from build123d import *

# Parameters (mm, degrees)
AUFSATZ_LINEAR_AUSTRAGEN1_DEPTH = 113
AUFSATZ_LINEAR_START            = -1
SKIZZE1_4_R                     = 3
AUFSATZ_LINEAR_AUSTRAGEN2_DEPTH = 1
SCHNITT_LINEAR_AUSTRAGEN1_DEPTH = 1
SKIZZE3_W                       = 2.5
SKIZZE3_H                       = 11
SKIZZE3_W_2                     = 3.5
SKIZZE3_H_2                     = 6.5
SCHNITT_LINEAR_AUSTRAGEN2_DEPTH = 2


with BuildPart() as part:
    # Skizze1 → Aufsatz-Linear austragen1 (new body)
    with BuildSketch(Plane(origin=(0, 0, 0), x_dir=(1, 0, 0), z_dir=(0, 1, 0))):
        with BuildLine():
            Line((-15.125, 17.875), (15.125, 17.875))
            ThreePointArc((15.125, 17.875), (17.069543648, 17.069543648), (17.875, 15.125))
            Line((17.875, 15.125), (17.875, -15.125))
            ThreePointArc((17.875, -15.125), (17.069543648, -17.069543648), (15.125, -17.875))
            Line((15.125, -17.875), (-15.125, -17.875))
            ThreePointArc((-15.125, -17.875), (-17.069543648, -17.069543648), (-17.875, -15.125))
            Line((-17.875, -15.125), (-17.875, 15.125))
            ThreePointArc((-17.875, 15.125), (-17.069543648, 17.069543648), (-15.125, 17.875))
        make_face()
        with BuildLine():
            ThreePointArc((-15.125, 16.875), (-16.362436867, 16.362436867), (-16.875, 15.125))
            Line((-16.875, 15.125), (-16.875, -15.125))
            ThreePointArc((-16.875, -15.125), (-16.362436867, -16.362436867), (-15.125, -16.875))
            Line((-15.125, -16.875), (15.125, -16.875))
            ThreePointArc((15.125, -16.875), (16.362436867, -16.362436867), (16.875, -15.125))
            Line((16.875, -15.125), (16.875, 15.125))
            ThreePointArc((16.875, 15.125), (16.362436867, 16.362436867), (15.125, 16.875))
            Line((15.125, 16.875), (-15.125, 16.875))
        make_face(mode=Mode.SUBTRACT)
    extrude(amount=AUFSATZ_LINEAR_AUSTRAGEN1_DEPTH)

    # Skizze1_4 → Aufsatz-Linear austragen2 (add)
    with BuildSketch(Plane(origin=(0, 0, 0), x_dir=(1, 0, 0), z_dir=(0, 1, 0)).offset(AUFSATZ_LINEAR_START)):
        with BuildLine():
            Line((15.125, 17.875), (-15.125, 17.875))
            ThreePointArc((-15.125, 17.875), (-17.069543648, 17.069543648), (-17.875, 15.125))
            Line((-17.875, 15.125), (-17.875, -15.125))
            ThreePointArc((-17.875, -15.125), (-17.069543648, -17.069543648), (-15.125, -17.875))
            Line((-15.125, -17.875), (15.125, -17.875))
            ThreePointArc((15.125, -17.875), (17.069543648, -17.069543648), (17.875, -15.125))
            Line((17.875, -15.125), (17.875, 15.125))
            ThreePointArc((17.875, 15.125), (17.069543648, 17.069543648), (15.125, 17.875))
        make_face()
        with BuildLine():
            Line((-10, 8), (10, 8))
            ThreePointArc((10, 8), (11.414213562, 7.414213562), (12, 6))
            Line((12, 6), (12, 0))
            ThreePointArc((12, 0), (11.414213562, -1.414213562), (10, -2))
            Line((10, -2), (-10, -2))
            ThreePointArc((-10, -2), (-11.414213562, -1.414213562), (-12, 0))
            Line((-12, 0), (-12, 6))
            ThreePointArc((-12, 6), (-11.414213562, 7.414213562), (-10, 8))
        make_face(mode=Mode.SUBTRACT)
        with Locations(Location((0, -9.5, 0), (0, 0, 270))):
            Circle(SKIZZE1_4_R, mode=Mode.SUBTRACT)
    extrude(amount=AUFSATZ_LINEAR_AUSTRAGEN2_DEPTH)

    # Skizze2 → Schnitt-Linear austragen1 (cut)
    with BuildSketch(Plane.XY.offset(17.875)):
        with BuildLine():
            Line((-10.5, 38), (10.5, 38))
            ThreePointArc((10.5, 38), (11.914213562, 37.414213562), (12.5, 36))
            Line((12.5, 36), (12.5, 27))
            ThreePointArc((12.5, 27), (11.914213562, 25.585786438), (10.5, 25))
            Line((10.5, 25), (-10.5, 25))
            ThreePointArc((-10.5, 25), (-11.914213562, 25.585786438), (-12.5, 27))
            Line((-12.5, 27), (-12.5, 36))
            ThreePointArc((-12.5, 36), (-11.914213562, 37.414213562), (-10.5, 38))
        make_face()
    extrude(amount=-SCHNITT_LINEAR_AUSTRAGEN1_DEPTH, mode=Mode.SUBTRACT)

    # Skizze3 → Schnitt-Linear austragen2 (cut)
    with BuildSketch(Plane(origin=(17.875, 0, 0), x_dir=(0, 0, -1), z_dir=(1, 0, 0))):
        with Locations((12.25, 7.5)):
            Rectangle(SKIZZE3_W, SKIZZE3_H)
        with Locations((13.75, 20.25)):
            Rectangle(SKIZZE3_W_2, SKIZZE3_H_2)
    extrude(amount=-SCHNITT_LINEAR_AUSTRAGEN2_DEPTH, mode=Mode.SUBTRACT)


solid = part.part
Can you work these out from the model? Positions are in its coordinate system, mm. A direction names the side the tool comes from. Coordinates: 2 decimals unless noted, no trailing zeros. Write each loop counter-clockwise with the first axis right and the second up, starting at its lowest first coordinate (ties: lowest second). Pieces come first, ordered by that corner, then holes. Notation, with made-up numbers: M -10,10 L 2,10 A16 cw 2,36 Z; hole C 37,5.25 d10. An arc over 180 degrees is marked long. Use one line per item in the form item = value.
Q1. For P1, Ø7, axis at x = 0, z = 9.5, coming from the +Y side; P2, Ø1.1, axis at x = 17.5, y = 18.5, coming from the -Z side; P3, Ø0.5, axis at x = 17.5, y = 6, coming from the +Z side; P4, Ø2, axis at x = -8, z = -6.5, coming from the -Y side, each with a flat end and sliding along its axis, tell me the tip position at first contact or that it passes through.
Model answer:
P1 = 0
P2 = -17.18
P3 = 16.87
P4 = through
Q2. If we section it at C-C (z = -4): Write out the boundary of the cut face in (x, y) (3 decimals), then the cut area to 3 significant figures.
Model answer:
outline = M -17.875,-1 L -12,-1 L -12,0 L -16.875,0 L -16.875,113 L -17.875,113 Z; M 12,-1 L 17.875,-1 L 17.875,113 L 16.875,113 L 16.875,0 L 12,0 Z
area = 238 mm^2
Q3. If we section it at D-D (x = 0): Write out the boundary of the cut face in (y, z) (3 decimals).
Model answer:
outline = M -1,-17.875 L 113,-17.875 L 113,-16.875 L 0,-16.875 L 0,-8 L -1,-8 Z; M -1,2 L 0,2 L 0,6.5 L -1,6.5 Z; M -1,12.5 L 0,12.5 L 0,16.875 L 25,16.875 L 25,17.875 L -1,17.875 Z; M 38,16.875 L 113,16.875 L 113,17.875 L 38,17.875 Z
Q4. We'd pull the mould along Z, two halves only. Please class faces 1 (the flat face through (16.875, 56, 0)), 2 (the cylindrical face through (11.9, 37.43, 17.38)), 3 (the cylindrical face through (-17.05, 55.2, -17.09)): +Z half, -Z half, draft (parallel to the pull), parting line (faces both ways), or undercut.
Model answer:
face_1 = undercut
face_2 = draft
face_3 = -Z half
Q5. If we section it at A-A (x = -7.5): Write out the boundary of the cut face in (y, z) (3 decimals), then the cut area to 3 significant figures.
Model answer:
outline = M -1,-17.875 L 113,-17.875 L 113,-16.875 L 0,-16.875 L 0,-8 L -1,-8 Z; M -1,2 L 0,2 L 0,16.875 L 25,16.875 L 25,17.875 L -1,17.875 Z; M 38,16.875 L 113,16.875 L 113,17.875 L 38,17.875 Z
area = 239 mm^2
Q6. If we section it at B-B (y = 44): Write out the boundary of the cut face in (x, z) (3 decimals).
Model answer:
outline = M -17.875,-15.125 A2.75 ccw -15.125,-17.875 L 15.125,-17.875 A2.75 ccw 17.875,-15.125 L 17.875,15.125 A2.75 ccw 15.125,17.875 L -15.125,17.875 A2.75 ccw -17.875,15.125 Z; hole M -16.875,-15.125 A1.75 ccw -15.125,-16.875 L 15.125,-16.875 A1.75 ccw 16.875,-15.125 L 16.875,15.125 A1.75 ccw 15.125,16.875 L -15.125,16.875 A1.75 ccw -16.875,15.125 Z
Q7. I need wall thicknesses on line 1 along Z through (x, y) = (-1, 10) (3 decimals); line 2 along X through (y, z) = (-0.8, 9.5) (3 decimals). Which ranges of each line are inside material? Lowest first, please. Write a range as from..to.
Model answer:
line_1 = -17.875..-16.875, 16.875..17.875
line_2 = -17.875..-3, 3..17.875
Q8. For faces 4 (the flat face through (0, 56, -16.875)), 5 (the cylindrical face through (11.43, -0.51, 1.4)), 6 (the cylindrical face through (-11.9, 25.57, 17.38)), which set-ups out of +Z, -Z, +X, -X, +Y, -Y let a thin tool reach every point of the face, with its end or its side?
Model answer:
face_4 = +Y
face_5 = +Y, -Y
face_6 = +Z
